from build123d import *

# Parameters (mm, degrees)
EXTRUDE_1_DEPTH     = 2
EXTRUDE_START       = 10.1
EXTRUDE_2_DEPTH     = 10.1
SKETCH_3_R          = 1.5
CUT_EXTRUDE_1_DEPTH = 228.860936532
EXTRUDE_START_2     = 3.5
SKETCH_6_R          = 4.5
SKETCH_6_R_2        = 1.5
EXTRUDE_3_DEPTH     = 3.5
SKETCH_7_W          = 15
SKETCH_7_H          = 7
CUT_EXTRUDE_2_DEPTH = 3


with BuildPart() as part:
    # Sketch 1 → Extrude 1 (new body)
    with BuildSketch(Plane(origin=(0, 0, 0), x_dir=(1, 0, 0), z_dir=(0, 1, 0))):
        with BuildLine():
            Line((197, 3), (3, 3))
            ThreePointArc((3, 3), (-1.242640687, 1.242640687), (-3, -3))
            Line((-3, -3), (-3, -47.100513143))
            ThreePointArc((-3, -47.100513143), (-2.32247943, -50.732097147), (-0.794949231, -54.09573922))
            Line((-0.794949231, -54.09573922), (30.796891429, -99.226940163))
            ThreePointArc((30.796891429, -99.226940163), (33.932268231, -102.05074496), (38.04363979, -103))
            Line((38.04363979, -103), (161.95636021, -103))
            ThreePointArc((161.95636021, -103), (166.067731769, -102.05074496), (169.203108571, -99.226940163))
            Line((169.203108571, -99.226940163), (200.794949231, -54.09573922))
            ThreePointArc((200.794949231, -54.09573922), (202.32247943, -50.732097147), (203, -47.100513143))
            Line((203, -47.100513143), (203, -3))
            ThreePointArc((203, -3), (201.242640687, 1.242640687), (197, 3))
        make_face()
    extrude(amount=-EXTRUDE_1_DEPTH)

    # Sketch 1_3 → Extrude 2 (add)
    with BuildSketch(Plane(origin=(0, 0, 0), x_dir=(1, 0, 0), z_dir=(0, 1, 0)).offset(EXTRUDE_START)):
        with BuildLine():
            Line((197, 3), (3, 3))
            ThreePointArc((3, 3), (-1.242640687, 1.242640687), (-3, -3))
            Line((-3, -3), (-3, -47.100513143))
            ThreePointArc((-3, -47.100513143), (-2.32247943, -50.732097147), (-0.794949231, -54.09573922))
            Line((-0.794949231, -54.09573922), (30.796891429, -99.226940163))
            ThreePointArc((30.796891429, -99.226940163), (33.932268231, -102.05074496), (38.04363979, -103))
            Line((38.04363979, -103), (161.95636021, -103))
            ThreePointArc((161.95636021, -103), (166.067731769, -102.05074496), (169.203108571, -99.226940163))
            Line((169.203108571, -99.226940163), (200.794949231, -54.09573922))
            ThreePointArc((200.794949231, -54.09573922), (202.32247943, -50.732097147), (203, -47.100513143))
            Line((203, -47.100513143), (203, -3))
            ThreePointArc((203, -3), (201.242640687, 1.242640687), (197, 3))
        make_face()
        with BuildLine():
            Line((0, -3), (0, -47))
            ThreePointArc((0, -47), (0.538734236, -49.830178992), (1.720387033, -52.457695762))
            Line((1.720387033, -52.457695762), (33.279612967, -97.542304238))
            ThreePointArc((33.279612967, -97.542304238), (35.317699373, -99.389808931), (38, -100))
            Line((38, -100), (162, -100))
            ThreePointArc((162, -100), (164.682300627, -99.389808931), (166.720387033, -97.542304238))
            Line((166.720387033, -97.542304238), (198.279612967, -52.457695762))
            ThreePointArc((198.279612967, -52.457695762), (199.461265764, -49.830178992), (200, -47))
            Line((200, -47), (200, -3))
            ThreePointArc((200, -3), (199.121320344, -0.878679656), (197, 0))
            Line((197, 0), (3, 0))
            ThreePointArc((3, 0), (0.878679656, -0.878679656), (0, -3))
        make_face(mode=Mode.SUBTRACT)
    extrude(amount=-EXTRUDE_2_DEPTH)

    # Sketch 3 → Cut-Extrude 1 (cut, through all)
    with BuildSketch(Plane(origin=(0, 0, 0), x_dir=(1, 0, 0), z_dir=(0, 1, 0))):
        with Locations(Location((45, -10, 0), (0, 0, 270))):
            Circle(SKETCH_3_R)
        with Locations(Location((20, -50, 0), (0, 0, 270))):
            Circle(SKETCH_3_R)
        with Locations(Location((35, -80, 0), (0, 0, 270))):
            Circle(SKETCH_3_R)
        with Locations(Location((85, -65, 0), (0, 0, 270))):
            Circle(SKETCH_3_R)
        with Locations(Location((155, -10, 0), (0, 0, 270))):
            Circle(SKETCH_3_R)
        with Locations(Location((180, -50, 0), (0, 0, 270))):
            Circle(SKETCH_3_R)
        with Locations(Location((165, -80, 0), (0, 0, 270))):
            Circle(SKETCH_3_R)
        with Locations(Location((115, -65, 0), (0, 0, 270))):
            Circle(SKETCH_3_R)
    extrude(amount=-CUT_EXTRUDE_1_DEPTH, mode=Mode.SUBTRACT)

    # Sketch 6 → Extrude 3 (add)
    # profile 1 of 8: a face of its own
    with BuildSketch(Plane(origin=(0, 0, 0), x_dir=(1, 0, 0), z_dir=(0, 1, 0)).offset(EXTRUDE_START_2)):
        with Locations(Location((85, -65, 0), (0, 0, 270))):
            Circle(SKETCH_6_R)
        with Locations(Location((85, -65, 0), (0, 0, 270))):
            Circle(SKETCH_6_R_2, mode=Mode.SUBTRACT)
    # profile 2 of 8: a face of its own
    with BuildSketch(Plane(origin=(0, 0, 0), x_dir=(1, 0, 0), z_dir=(0, 1, 0)).offset(EXTRUDE_START_2)):
        with Locations(Location((35, -80, 0), (0, 0, 270))):
            Circle(SKETCH_6_R)
        with Locations(Location((35, -80, 0), (0, 0, 270))):
            Circle(SKETCH_6_R_2, mode=Mode.SUBTRACT)
    # profile 3 of 8: a face of its own
    with BuildSketch(Plane(origin=(0, 0, 0), x_dir=(1, 0, 0), z_dir=(0, 1, 0)).offset(EXTRUDE_START_2)):
        with Locations(Location((20, -50, 0), (0, 0, 270))):
            Circle(SKETCH_6_R)
        with Locations(Location((20, -50, 0), (0, 0, 270))):
            Circle(SKETCH_6_R_2, mode=Mode.SUBTRACT)
    # profile 4 of 8: a face of its own
    with BuildSketch(Plane(origin=(0, 0, 0), x_dir=(1, 0, 0), z_dir=(0, 1, 0)).offset(EXTRUDE_START_2)):
        with Locations(Location((45, -10, 0), (0, 0, 270))):
            Circle(SKETCH_6_R)
        with Locations(Location((45, -10, 0), (0, 0, 270))):
            Circle(SKETCH_6_R_2, mode=Mode.SUBTRACT)
    # profile 5 of 8: a face of its own
    with BuildSketch(Plane(origin=(0, 0, 0), x_dir=(1, 0, 0), z_dir=(0, 1, 0)).offset(EXTRUDE_START_2)):
        with Locations(Location((155, -10, 0), (0, 0, 270))):
            Circle(SKETCH_6_R)
        with Locations(Location((155, -10, 0), (0, 0, 270))):
            Circle(SKETCH_6_R_2, mode=Mode.SUBTRACT)
    # profile 6 of 8: a face of its own
    with BuildSketch(Plane(origin=(0, 0, 0), x_dir=(1, 0, 0), z_dir=(0, 1, 0)).offset(EXTRUDE_START_2)):
        with Locations(Location((115, -65, 0), (0, 0, 270))):
            Circle(SKETCH_6_R)
        with Locations(Location((115, -65, 0), (0, 0, 270))):
            Circle(SKETCH_6_R_2, mode=Mode.SUBTRACT)
    # profile 7 of 8: a face of its own
    with BuildSketch(Plane(origin=(0, 0, 0), x_dir=(1, 0, 0), z_dir=(0, 1, 0)).offset(EXTRUDE_START_2)):
        with Locations(Location((180, -50, 0), (0, 0, 270))):
            Circle(SKETCH_6_R)
        with Locations(Location((180, -50, 0), (0, 0, 270))):
            Circle(SKETCH_6_R_2, mode=Mode.SUBTRACT)
    # profile 8 of 8: a face of its own
    with BuildSketch(Plane(origin=(0, 0, 0), x_dir=(1, 0, 0), z_dir=(0, 1, 0)).offset(EXTRUDE_START_2)):
        with Locations(Location((165, -80, 0), (0, 0, 270))):
            Circle(SKETCH_6_R)
        with Locations(Location((165, -80, 0), (0, 0, 270))):
            Circle(SKETCH_6_R_2, mode=Mode.SUBTRACT)
    extrude(amount=-EXTRUDE_3_DEPTH)

    # Sketch 7 → Cut-Extrude 2 (cut)
    with BuildSketch(Plane(origin=(0, 0, -3), x_dir=(-1, 0, 0), z_dir=(0, 0, -1))):
        with Locations((-100, 1.5)):
            Rectangle(SKETCH_7_W, SKETCH_7_H)
    extrude(amount=-CUT_EXTRUDE_2_DEPTH, mode=Mode.SUBTRACT)


solid = part.part
Check sheet for the modelled part. Datum: model origin and axes. Units: mm. A direction names the side the tool comes from. Give positions to 0.01 mm unless a question says otherwise; leave off trailing zeros. Write each loop counter-clockwise with the first axis right and the second up, starting at its lowest first coordinate (ties: lowest second). Pieces come first, ordered by that corner, then holes. Notation, with made-up numbers: (41, -30) -> (46, -30) arc R14 ccw to (46, -3) -> close; hole circle Ø7 at (-10.75, -37). An arc over 180 degrees is marked (long way). Write item = value, one per line.
Item 1: Release check for a two-part mould opening along Z. For faces 3 (the flat face through (184.778, 4.135, 76.977)), 4 (the flat face through (18, 3.5, 50)), 5 (the flat face through (100, 10.1, -1)) record: +Z half, -Z half, draft (parallel to the pull), parting line (faces both ways), or undercut.
Output:
face_3 = +Z half
face_4 = undercut
face_5 = draft
Item 2: Tool access check on faces 1 (the flat face through (115, 3.5, 67)), 2 (the flat face through (101.4, 5.5, -3)). Record the directions out of +Z, -Z, +X, -X, +Y, -Y that give a thin tool (end or side, any length) a straight path to the whole face; none if there is none.
Output:
face_1 = +Y
face_2 = -Z, +X, -X, +Y, -Y
Item 3: Sectioned sample at A-A on x = 94.5. Record the boundary of the cut face in (y, z), and give its area (3 significant figures).
Output:
outline = (-2, 0) -> (0, 0) -> (0, 100) -> (10.1, 100) -> (10.1, 103) -> (-2, 103) -> close; (5, -3) -> (10.1, -3) -> (10.1, 0) -> (5, 0) -> close
area = 252 mm^2
Item 4: Sectioned sample at B-B on y = 7.5. Record the boundary of the cut face in (x, z).
Output:
outline = (-3, 3) arc R6 ccw to (3, -3) -> (197, -3) arc R6 ccw to (203, 3) -> (203, 47.1) arc R15.31 ccw to (200.79, 54.1) -> (169.2, 99.23) arc R8.42 ccw to (161.96, 103) -> (38.04, 103) arc R8.42 ccw to (30.8, 99.23) -> (-0.79, 54.1) arc R15.31 ccw to (-3, 47.1) -> close; hole (0, 3) arc R3 ccw to (3, 0) -> (197, 0) arc R3 ccw to (200, 3) -> (200, 47) arc R12.31 ccw to (198.28, 52.46) -> (166.72, 97.54) arc R5.42 ccw to (162, 100) -> (38, 100) arc R5.42 ccw to (33.28, 97.54) -> (1.72, 52.46) arc R12.31 ccw to (0, 47) -> close
Item 5: Sectioned sample at D-D on z = 71.5. Record the boundary of the cut face in (x, y).
Output:
outline = (11.39, -2) -> (188.61, -2) -> (188.61, 10.1) -> (184.95, 10.1) -> (184.95, 0) -> (15.05, 0) -> (15.05, 10.1) -> (11.39, 10.1) -> close
Item 6: Sectioned sample at C-C on x = 122.5. Record the boundary of the cut face in (y, z).
Output:
outline = (-2, -3) -> (10.1, -3) -> (10.1, 0) -> (0, 0) -> (0, 100) -> (10.1, 100) -> (10.1, 103) -> (-2, 103) -> close
Item 7: Gauge pin test, flat ends, axial feed: pin 1 (4.5 mm diameter, centred on x = 20.5, z = 49.5, fed in from +Y); pin 2 (2 mm diameter, centred on x = 99, y = -1, fed in from -Z); pin 3 (4 mm diameter, centred on x = 122, z = 89, fed in from +Y). Record the tip position at first contact, or that the pin passes through.
Output:
pin_1 = 3.5
pin_2 = 0
pin_3 = 0
Item 8: Scan lines: probe 1 along X at (y, z) = (9, 19); probe 2 along Z at (x, y) = (62.5, 4.25); probe 3 along Z at (x, y) = (85, -0.7). Record each from-to range of solid material in increasing order. Write a range as from..to.
Output:
probe_1 = -3..0, 200..203
probe_2 = -3..0, 100..103
probe_3 = -3..63.5, 66.5..103
